from build123d import *

# Parameters (mm, degrees)
F0_W     = 0.3
F0_H     = 3.8
F0_W_2   = 0.6
F0_H_2   = 0.6
F1_DEPTH = 0.6


with BuildPart() as f1:
    # F0 (on Front) → F1 (new body)
    with BuildSketch(Plane.XZ):
        with Locations((-0.15, 2.5)):
            Rectangle(F0_W, F0_H)
        with Locations((-7.8, 0.3)):
            Rectangle(F0_W_2, F0_H_2)
        with Locations((-7.8, 2.5)):
            Rectangle(F0_W_2, F0_H)
        Polygon((0, 5), (0, 4.4), (0.3, 4.4), (3.75, 4.4), (4.35, 4.4), (7.5, 4.4), (7.5, 5), align=None)
        Polygon((-0.3, 4.4), (0, 4.4), (0, 5), (-7.5, 5), (-7.5, 4.4), (-4.35, 4.4), (-3.75, 4.4), align=None)
        with Locations((0.15, 2.5)):
            Rectangle(F0_W, F0_H)
        with Locations((4.05, 2.5)):
            Rectangle(F0_W_2, F0_H)
        with Locations((7.8, 2.5)):
            Rectangle(F0_W_2, F0_H)
        with Locations((-7.8, 4.7)):
            Rectangle(F0_W_2, F0_H_2)
        Polygon((-7.5, 0), (0, 0), (0, 0.6), (-0.3, 0.6), (-3.75, 0.6), (-4.35, 0.6), (-7.5, 0.6), align=None)
        with Locations((7.8, 0.3)):
            Rectangle(F0_W_2, F0_H_2)
        with Locations((-4.05, 2.5)):
            Rectangle(F0_W_2, F0_H)
        Polygon((0, 0.6), (0, 0), (7.5, 0), (7.5, 0.6), (4.35, 0.6), (3.75, 0.6), (0.3, 0.6), align=None)
        with Locations((7.8, 4.7)):
            Rectangle(F0_W_2, F0_H_2)
    extrude(amount=F1_DEPTH)


solid = f1.part
Geometry check sheet. Reference: the model listing, model coordinates, mm. Give positions to 0.01 mm unless a question says otherwise; leave off trailing zeros. Loops run counter-clockwise (first coordinate to the right, second up) from the corner with the lowest first, then second, coordinate; pieces in that order, holes last. Notation, with made-up numbers: M 41.5,70.5 L 68.5,70.5 A26 ccw 68.5,85.5 Z; hole C -40,76.5 d5. An arc over 180 degrees is marked long. Write each question's results on one line, items separated by ' | '.
1) Section check B-B, the plane z = 1.85. Record the boundary of the cut face in (x, y), plus the area to 3 significant figures.
Answers follow:
outline: M -8.1,-0.6 L -7.5,-0.6 L -7.5,0 L -8.1,0 Z; M -4.35,-0.6 L -3.75,-0.6 L -3.75,0 L -4.35,0 Z; M -0.3,-0.6 L 0.3,-0.6 L 0.3,0 L -0.3,0 Z; M 3.75,-0.6 L 4.35,-0.6 L 4.35,0 L 3.75,0 Z; M 7.5,-0.6 L 8.1,-0.6 L 8.1,0 L 7.5,0 Z | area: 1.80 mm2
2) Section check A-A, the plane x = 7. Record the boundary of the cut face in (y, z).
Answers follow:
outline: M -0.6,0 L 0,0 L 0,0.6 L -0.6,0.6 Z; M -0.6,4.4 L 0,4.4 L 0,5 L -0.6,5 Z
3) Section check C-C, the plane y = -0.15. Record the boundary of the cut face in (x, z), plus the area to 3 significant figures.
Answers follow:
outline: M -8.1,0 L 8.1,0 L 8.1,5 L -8.1,5 Z; hole M -7.5,0.6 L -4.35,0.6 L -4.35,4.4 L -7.5,4.4 Z; hole M -3.75,0.6 L -0.3,0.6 L -0.3,4.4 L -3.75,4.4 Z; hole M 0.3,0.6 L 3.75,0.6 L 3.75,4.4 L 0.3,4.4 Z; hole M 4.35,0.6 L 7.5,0.6 L 7.5,4.4 L 4.35,4.4 Z | area: 30.8 mm2
4) Thickness scan on line 1 (X direction, y = -0.35, z = 3.5); line 2 (Z direction, x = -7, y = -0.25). Record the ranges inside material, lowest first.
Answers follow:
line 1: -8.1 to -7.5, -4.35 to -3.75, -0.3 to 0.3, 3.75 to 4.35, 7.5 to 8.1 | line 2: 0 to 0.6, 4.4 to 5
